```python
from build123d import *

# Parameters (mm, degrees)
ESQUISSE2_R             = 2
BOSS_EXTRU_1_DEPTH      = 14
ENL_V_MAT_EXTRU_1_DEPTH = 7


with BuildPart() as part:
    # Esquisse1 → Révolution1 (revolve)
    with BuildSketch(Plane.XY, mode=Mode.PRIVATE) as r_volution1_sk:
        with BuildLine():
            Line((-7.250462296, 3.380946094), (-5.437846722, 2.53570957))
            ThreePointArc((-5.437846722, 2.53570957), (-5.060348675, -3.22379765), (0, -6))
            Line((0, -6), (0, -8))
            ThreePointArc((0, -8), (-6.747131567, -4.298396867), (-7.250462296, 3.380946094))
        make_face()
    revolve(r_volution1_sk.sketch.rotate(Axis((0, 0, 0), (0, -1, 0)), 270), axis=Axis((0, 0, 0), (0, -1, 0)))

    # Esquisse2 → Boss.-Extru.1 (add)
    with BuildSketch(Plane(origin=(0, 0, 0), x_dir=(1, 0, 0), z_dir=(0, 1, 0))):
        with Locations(Location((0, 0, 0), (0, 0, 270))):
            Circle(ESQUISSE2_R)
    extrude(amount=-BOSS_EXTRU_1_DEPTH)

    # Esquisse3 → Enlèv. mat.-Extru.1 (cut)
    with BuildSketch(Plane(origin=(-10.393608687, -1.299249719, -2.818585808), x_dir=(-0.25784022856565836, -0.03223123504955077, 0.9656498143842775), z_dir=(-0.9581923956348063, -0.11977853300162247, -0.2598469472201095))):
        with BuildLine():
            Line((-4, 2), (4, 2))
            ThreePointArc((4, 2), (6, 0), (4, -2))
            Line((4, -2), (-4, -2))
            ThreePointArc((-4, -2), (-6, 0), (-4, 2))
        make_face()
    extrude(amount=-ENL_V_MAT_EXTRU_1_DEPTH, mode=Mode.SUBTRACT)


solid = part.part
```
Geometry check sheet. Reference: the model listing, model coordinates, mm. A direction names the side the tool comes from. Give positions to 0.01 mm unless a question says otherwise; leave off trailing zeros. Write each loop counter-clockwise with the first axis right and the second up, starting at its lowest first coordinate (ties: lowest second). Pieces come first, ordered by that corner, then holes.
1) Gauge pin test, flat ends, axial feed: pin 1 (1 mm diameter, centred on x = -3, z = 3.5, fed in from -Y); pin 2 (8 mm diameter, centred on y = -9, z = -3.5, fed in from -X); pin 3 (2 mm diameter, centred on x = 0.5, z = 0.5, fed in from +Y). Record the tip position at first contact, or that the pin passes through.
2) Section check B-B, the plane y = -4.5. Record the boundary of the cut face in (x, z), and give its area (3 significant figures).
3) Access from +Z, -Z, +X, -X, +Y, -Y to the whole of each face (thin tool, end or side, straight path). Record for faces 1 (the flat face through (-5.818, -2.743, -1.587)), 2 (the cylindrical face through (-2, -3, 0)), 3 (the flat face through (-6.29, 1.23, -1.7)).
4) Section check A-A, the plane z = 0. Record the boundary of the cut face in (x, y), and give its area (3 significant figures).
5) Release check for a two-part mould opening along Z. For faces 4 (the cylindrical face through (-2, -11, 0)), 5 (the cylindrical face through (-3.19, -0.44, -7.08)), 6 (the flat face through (0, -14, 0)) record: pulls with the +Z half, pulls with the -Z half, needs draft (parallel to the pull), parting line crosses it, or undercut.
6) Section check D-D, the plane y = -8.5. Record the boundary of the cut face in (x, z), and give its area (3 significant figures).
7) Section check C-C, the plane x = 0. Record the boundary of the cut face in (y, z).
8) Material ranges on L1, parallel to Z at x = 0.25, y = -3; L2, parallel to Y at x = -1, z = 1.5; L3, parallel to Z at x = 4, y = 1.75, recorded low to high.
Computed:
1. pin 1: stops at y = -6.86
1. pin 2: stops at x = -5.66
1. pin 3: stops at y = 0
2. outline: circle Ø13.23 at (0, 0); circle Ø4 at (0, 0); hole circle Ø7.94 at (0, 0)
2. area: 101 mm2
3. face 1: -X
3. face 2: +Y
3. face 3: none
4. outline: (-7.93, 1.02) - (-5.86, 1.28) arc R6 cw to (-5.44, 2.54) - (-7.25, 3.38) arc R8 ccw to start; (-7.44, -2.95) arc R8 ccw to (-2, -7.75) - (-2, -14) - (2, -14) - (2, -7.75) arc R8 ccw to (7.25, 3.38) - (5.44, 2.54) arc R6 cw to (2, -5.66) - (2, 0) - (-2, 0) - (-2, -5.66) arc R6 cw to (-5.37, -2.69) - close
4. area: 96.0 mm2
5. face 4: parting line crosses it
5. face 5: undercut
5. face 6: needs draft
6. outline: circle Ø4 at (0, 0)
6. area: 12.6 mm2
7. outline: (-14, -2) - (-7.75, -2) arc R8 ccw to (3.38, -7.25) - (2.54, -5.44) arc R6 cw to (-5.66, -2) - (0, -2) - (0, 2) - (-5.66, 2) arc R6 cw to (2.54, 5.44) - (3.38, 7.25) arc R8 ccw to (-7.75, 2) - (-14, 2) - close
8. L1: z = -7.41 to -5.19, -1.98 to 1.98, 5.19 to 7.41
8. L2: y = -14 to 0
8. L3: z = -6.7 to -4.12, 4.12 to 6.7
